from build123d import *

# Parameters (mm, degrees)
EXTRUDE_1_DEPTH     = 4
SKETCH_3_R          = 2.1
CUT_EXTRUDE_1_DEPTH = 10


with BuildPart() as part:
    # 草图2 → 凸台-拉伸1 (new body)
    with BuildSketch(Plane(origin=(0, 0, 0), x_dir=(0, 0, -1), z_dir=(1, 0, 0))):
        with BuildLine():
            Line((-211.25, 80.041666667), (-171.25, 80.041666667))
            ThreePointArc((-171.25, 80.041666667), (-169.128679656, 79.16298701), (-168.25, 77.041666667))
            Line((-168.25, 77.041666667), (-168.25, 33.041666667))
            ThreePointArc((-168.25, 33.041666667), (-169.128679656, 30.920346323), (-171.25, 30.041666667))
            Line((-171.25, 30.041666667), (-185.25, 30.041666667))
            ThreePointArc((-185.25, 30.041666667), (-187.371320344, 30.920346323), (-188.25, 33.041666667))
            Line((-188.25, 33.041666667), (-188.25, 54.041666667))
            ThreePointArc((-188.25, 54.041666667), (-190.007359313, 58.284307354), (-194.25, 60.041666667))
            Line((-194.25, 60.041666667), (-211.25, 60.041666667))
            ThreePointArc((-211.25, 60.041666667), (-213.371320344, 60.920346323), (-214.25, 63.041666667))
            Line((-214.25, 63.041666667), (-214.25, 77.041666667))
            ThreePointArc((-214.25, 77.041666667), (-213.371320344, 79.16298701), (-211.25, 80.041666667))
        make_face()
    extrude(amount=EXTRUDE_1_DEPTH)

    # 草图3 → 切除-拉伸1 (cut)
    with BuildSketch(Plane(origin=(4, 0, 0), x_dir=(0, 0, -1), z_dir=(1, 0, 0))):
        with Locations((-208.25, 70.041666667)):
            Circle(SKETCH_3_R)
        with Locations((-178.25, 70.041666667)):
            Circle(SKETCH_3_R)
        with Locations((-178.25, 39.041666667)):
            Circle(SKETCH_3_R)
        with Locations((-196.25, 70.041666667)):
            Circle(SKETCH_3_R)
    extrude(amount=-CUT_EXTRUDE_1_DEPTH, mode=Mode.SUBTRACT)


solid = part.part
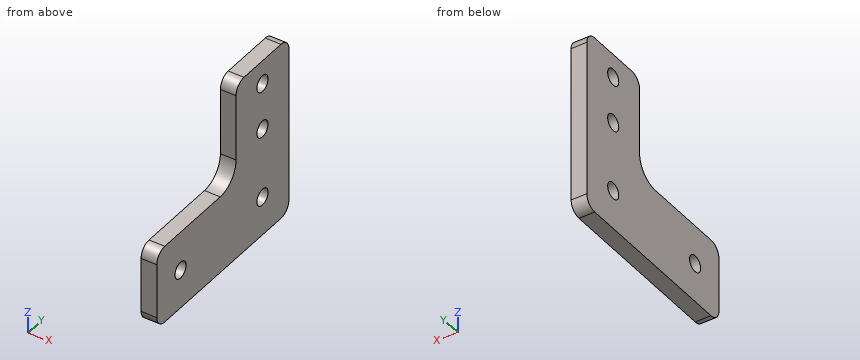
Build history of the part. All positions in model axes, mm. Coordinates: 2 decimals unless noted, no trailing zeros. Order: outer loops, then holes, each group sorted by start corner. A loop starts at its lowest first (then second) coordinate and runs counter-clockwise, first axis right, second up. Notation, with made-up numbers: (6, 35) - (48, 35) arc R21 cw to (48, 61) - close; hole circle Ø10 at (63, 50). An arc over 180 degrees is marked (long way). Write each question's results on one line, items separated by ' | '. Start each with the question number.
Item 1: Flat gauge pins, fed straight in: pin 1 (2 mm diameter, centred on x = 2.5, z = 187, fed in from -Y); pin 2 (10 mm diameter, centred on y = 53, z = 198, fed in from +X); pin 3 (2 mm diameter, centred on x = 1.5, z = 206, fed in from -Y). Where does each tip first touch, or does it go through?
Item 2: Band-saw the part on D-D on x = 2. Write the cut outline in (y, z).
Item 3: Band-saw the part on C-C on y = 53. Write the cut outline in (x, z).
Item 4: Band-saw the part on A-A on z = 178.25. Write the cut outline in (x, y), and give its area (3 significant figures).
Item 5: Band-saw the part on B-B on z = 208.25. Write the cut outline in (x, y), and give its area (3 significant figures).
Item 6: Wall check: probe 1 along Y at (x, z) = (2.7, 178.25); probe 2 along Y at (x, z) = (3.05, 196.25); probe 3 along Y at (x, z) = (1.35, 177). Give the ranges that are in metal, low to high. Write a range as [from, to].
Numbers:
1) pin 1: y = 30.14 | pin 2: through | pin 3: y = 60.04
2) outline: (30.04, 171.25) arc R3 ccw to (33.04, 168.25) - (77.04, 168.25) arc R3 ccw to (80.04, 171.25) - (80.04, 211.25) arc R3 ccw to (77.04, 214.25) - (63.04, 214.25) arc R3 ccw to (60.04, 211.25) - (60.04, 194.25) arc R6 cw to (54.04, 188.25) - (33.04, 188.25) arc R3 ccw to (30.04, 185.25) - close; hole circle Ø4.2 at (39.04, 178.25); hole circle Ø4.2 at (70.04, 178.25); hole circle Ø4.2 at (70.04, 196.25); hole circle Ø4.2 at (70.04, 208.25)
3) outline: (0, 168.25) - (4, 168.25) - (4, 188.25) - (0, 188.25) - close
4) outline: (0, 30.04) - (4, 30.04) - (4, 36.94) - (0, 36.94) - close; (0, 41.14) - (4, 41.14) - (4, 67.94) - (0, 67.94) - close; (0, 72.14) - (4, 72.14) - (4, 80.04) - (0, 80.04) - close | area: 166 mm^2
5) outline: (0, 60.04) - (4, 60.04) - (4, 67.94) - (0, 67.94) - close; (0, 72.14) - (4, 72.14) - (4, 80.04) - (0, 80.04) - close | area: 63.2 mm^2
6) probe 1: [30.04, 36.94], [41.14, 67.94], [72.14, 80.04] | probe 2: [60.04, 67.94], [72.14, 80.04] | probe 3: [30.04, 37.35], [40.73, 68.35], [71.73, 80.04]
